```python
from build123d import *

# Parameters (mm, degrees)
IZIM1_W                               = 47
IZIM1_H                               = 96.3
Y_KSEKLIK_EKSTR_ZYON1_DEPTH           = 2
KES_EKSTR_ZYON1_DEPTH                 = 68.315841375
IZIM3_R                               = 3
Y_KSEKLIK_EKSTR_ZYON2_DEPTH           = 5
Y_KSEKLIK_EKSTR_ZYON3_DEPTH           = 2
Y_KSEKLIK_EKSTR_ZYON3_DRAFT           = 4
Y_KSEKLIK_EKSTR_ZYON3_PROFILE_2_DEPTH = 2
Y_KSEKLIK_EKSTR_ZYON3_PROFILE_2_DRAFT = 4
Y_KSEKLIK_EKSTR_ZYON3_PROFILE_3_DEPTH = 2
Y_KSEKLIK_EKSTR_ZYON3_PROFILE_3_DRAFT = 4
IZIM5_W                               = 47
IZIM5_H                               = 2.496748802
KES_EKSTR_ZYON3_DEPTH                 = 4
IZIM6_W                               = 4
IZIM6_H                               = 4
Y_KSEKLIK_EKSTR_ZYON4_DEPTH           = 6
IZIM7_R                               = 1.25
KES_EKSTR_ZYON4_DEPTH                 = 4
KES_EKSTR_ZYON4_DRAFT                 = -2
KES_EKSTR_ZYON4_PROFILE_2_DEPTH       = 4
KES_EKSTR_ZYON4_PROFILE_2_DRAFT       = -2
IZIM8_R                               = 1.25
Y_KSEKLIK_EKSTR_ZYON5_DEPTH           = 0.1
KUBBE5_FACE_RADIUS                    = 1.25
KUBBE5_HEIGHT                         = 1
AYNALAMA8_COPY_1_FACE_RADIUS          = 1.25
AYNALAMA8_COPY_1_HEIGHT               = 1


with BuildPart() as part:
    # Çizim1 → Yükseklik-Ekstrüzyon1 (new body)
    with BuildSketch(Plane(origin=(0, 0, 0), x_dir=(1, 0, 0), z_dir=(0, 1, 0))):
        Rectangle(IZIM1_W, IZIM1_H)
    extrude(amount=Y_KSEKLIK_EKSTR_ZYON1_DEPTH)

    # Çizim2 → Kes-Ekstrüzyon1 (cut, through all)
    with BuildSketch(Plane.ZY.offset(23.5)):
        Polygon((48.15, 0), (43.722619458, 2), (48.15, 2), align=None)
    extrude(amount=-KES_EKSTR_ZYON1_DEPTH, mode=Mode.SUBTRACT)

    # Çizim3 → Yükseklik-Ekstrüzyon2 (add)
    # profile 1 of 4: a face of its own
    with BuildSketch(Plane(origin=(0, 2, 0), x_dir=(1, 0, 0), z_dir=(0, 1, 0))):
        with Locations(Location((-15, 25.194528994, 0), (0, 0, 270))):
            Circle(IZIM3_R)
        with BuildLine():
            ThreePointArc((-16.5, 25.194528994), (-15, 23.694528994), (-13.5, 25.194528994))
            ThreePointArc((-13.5, 25.194528994), (-15, 26.694528994), (-16.5, 25.194528994))
        make_face(mode=Mode.SUBTRACT)
    # profile 2 of 4: a face of its own
    with BuildSketch(Plane(origin=(0, 2, 0), x_dir=(1, 0, 0), z_dir=(0, 1, 0))):
        with Locations(Location((15, 25.194528994, 0), (0, 0, 270))):
            Circle(IZIM3_R)
        with BuildLine():
            ThreePointArc((13.5, 25.194528994), (15, 23.694528994), (16.5, 25.194528994))
            ThreePointArc((16.5, 25.194528994), (15, 26.694528994), (13.5, 25.194528994))
        make_face(mode=Mode.SUBTRACT)
    # profile 3 of 4: a face of its own
    with BuildSketch(Plane(origin=(0, 2, 0), x_dir=(1, 0, 0), z_dir=(0, 1, 0))):
        with Locations(Location((-3.3, -16.805471006, 0), (0, 0, 270))):
            Circle(IZIM3_R)
        with BuildLine():
            ThreePointArc((-1.8, -16.805471006), (-3.3, -15.305471006), (-4.8, -16.805471006))
            ThreePointArc((-4.8, -16.805471006), (-3.3, -18.305471006), (-1.8, -16.805471006))
        make_face(mode=Mode.SUBTRACT)
    # profile 4 of 4: a face of its own
    with BuildSketch(Plane(origin=(0, 2, 0), x_dir=(1, 0, 0), z_dir=(0, 1, 0))):
        with Locations(Location((11.7, -16.805471006, 0), (0, 0, 270))):
            Circle(IZIM3_R)
        with BuildLine():
            ThreePointArc((10.2, -16.805471006), (11.7, -18.305471006), (13.2, -16.805471006))
            ThreePointArc((13.2, -16.805471006), (11.7, -15.305471006), (10.2, -16.805471006))
        make_face(mode=Mode.SUBTRACT)
    extrude(amount=Y_KSEKLIK_EKSTR_ZYON2_DEPTH)


with BuildPart() as y_kseklik_ekstr_zyon3_tool:
    # Çizim4 → Yükseklik-Ekstrüzyon3 (with draft: the straight prism first)
    with BuildSketch(Plane(origin=(0, 18.064663731, 8.160429654), x_dir=(1, 0, 0), z_dir=(0, 0.9113290688724396, 0.4116786710871625))):
        Polygon((20.223356646, -43.072925072), (18.923356646, -43.072925072), (19.573356646, -44.562410878), align=None)
    extrude(amount=Y_KSEKLIK_EKSTR_ZYON3_DEPTH)
    # Yükseklik-Ekstrüzyon3: the draft: its side faces are tilted about the plane it starts from
    y_kseklik_ekstr_zyon3_sides = [y_kseklik_ekstr_zyon3_tool.faces().sort_by_distance(p)[0] for p in [
        (19.573356646, 1.243788246, 47.825717025),
        (19.248356646, 0.937193478, 48.504422881),
        (19.898356646, 0.937193478, 48.504422881),
    ]]
    draft(y_kseklik_ekstr_zyon3_sides, Plane(origin=(0, 18.064663731, 8.160429654), x_dir=(1, 0, 0), z_dir=(0, 0.9113290688724396, 0.4116786710871625)), Y_KSEKLIK_EKSTR_ZYON3_DRAFT)


with BuildPart() as part_1:
    add(part.part)

    # Yükseklik-Ekstrüzyon3: add y_kseklik_ekstr_zyon3_tool
    add(y_kseklik_ekstr_zyon3_tool.part)


with BuildPart() as y_kseklik_ekstr_zyon3_profile_2_tool:
    # Çizim4 → Yükseklik-Ekstrüzyon3 profile 2 (with draft: the straight prism first)
    with BuildSketch(Plane(origin=(0, 18.064663731, 8.160429654), x_dir=(1, 0, 0), z_dir=(0, 0.9113290688724396, 0.4116786710871625))):
        Polygon((0.223356646, -43.072925072), (-1.076643354, -43.072925072), (-0.426643354, -44.562410878), align=None)
    extrude(amount=Y_KSEKLIK_EKSTR_ZYON3_PROFILE_2_DEPTH)
    # Yükseklik-Ekstrüzyon3 profile 2: the draft: its side faces are tilted about the plane it starts from
    y_kseklik_ekstr_zyon3_profile_2_sides = [y_kseklik_ekstr_zyon3_profile_2_tool.faces().sort_by_distance(p)[0] for p in [
        (-0.426643354, 1.243788246, 47.825717025),
        (-0.751643354, 0.937193478, 48.504422881),
        (-0.101643354, 0.937193478, 48.504422881),
    ]]
    draft(y_kseklik_ekstr_zyon3_profile_2_sides, Plane(origin=(0, 18.064663731, 8.160429654), x_dir=(1, 0, 0), z_dir=(0, 0.9113290688724396, 0.4116786710871625)), Y_KSEKLIK_EKSTR_ZYON3_PROFILE_2_DRAFT)


with BuildPart() as part_2:
    add(part_1.part)

    # Yükseklik-Ekstrüzyon3 profile 2: add y_kseklik_ekstr_zyon3_profile_2_tool
    add(y_kseklik_ekstr_zyon3_profile_2_tool.part)


with BuildPart() as y_kseklik_ekstr_zyon3_profile_3_tool:
    # Çizim4 → Yükseklik-Ekstrüzyon3 profile 3 (with draft: the straight prism first)
    with BuildSketch(Plane(origin=(0, 18.064663731, 8.160429654), x_dir=(1, 0, 0), z_dir=(0, 0.9113290688724396, 0.4116786710871625))):
        Polygon((-21.076643354, -43.072925072), (-20.426643354, -44.562410878), (-19.776643354, -43.072925072), align=None)
    extrude(amount=Y_KSEKLIK_EKSTR_ZYON3_PROFILE_3_DEPTH)
    # Yükseklik-Ekstrüzyon3 profile 3: the draft: its side faces are tilted about the plane it starts from
    y_kseklik_ekstr_zyon3_profile_3_sides = [y_kseklik_ekstr_zyon3_profile_3_tool.faces().sort_by_distance(p)[0] for p in [
        (-20.751643354, 0.937193478, 48.504422881),
        (-20.101643354, 0.937193478, 48.504422881),
        (-20.426643354, 1.243788246, 47.825717025),
    ]]
    draft(y_kseklik_ekstr_zyon3_profile_3_sides, Plane(origin=(0, 18.064663731, 8.160429654), x_dir=(1, 0, 0), z_dir=(0, 0.9113290688724396, 0.4116786710871625)), Y_KSEKLIK_EKSTR_ZYON3_PROFILE_3_DRAFT)


with BuildPart() as part_3:
    add(part_2.part)

    # Yükseklik-Ekstrüzyon3 profile 3: add y_kseklik_ekstr_zyon3_profile_3_tool
    add(y_kseklik_ekstr_zyon3_profile_3_tool.part)

    # Çizim5 → Kes-Ekstrüzyon3 (cut)
    with BuildSketch(Plane.XZ):
        with Locations((0, 49.398374401)):
            Rectangle(IZIM5_W, IZIM5_H)
    extrude(amount=KES_EKSTR_ZYON3_DEPTH, mode=Mode.SUBTRACT)

    # Çizim6 → Yükseklik-Ekstrüzyon4 (add)
    with BuildSketch(Plane(origin=(0, 2, 0), x_dir=(1, 0, 0), z_dir=(0, 1, 0))):
        with Locations((-21.5, 46.15)):
            Rectangle(IZIM6_W, IZIM6_H)
        with Locations((21.5, 46.15)):
            Rectangle(IZIM6_W, IZIM6_H)
        with Locations((-21.5, -23.85)):
            Rectangle(IZIM6_W, IZIM6_H)
        with Locations((21.5, -23.85)):
            Rectangle(IZIM6_W, IZIM6_H)
    extrude(amount=Y_KSEKLIK_EKSTR_ZYON4_DEPTH)


with BuildPart() as kes_ekstr_zyon4_tool:
    # Çizim7 → Kes-Ekstrüzyon4 (with draft: the straight prism first)
    with BuildSketch(Plane(origin=(0, 0, -48.15), x_dir=(-1, 0, 0), z_dir=(0, 0, -1))):
        with Locations((-21.5, 6)):
            Circle(IZIM7_R)
    extrude(amount=-KES_EKSTR_ZYON4_DEPTH)
    # Kes-Ekstrüzyon4: the draft: its side faces are tilted about the plane it starts from
    kes_ekstr_zyon4_sides = [kes_ekstr_zyon4_tool.faces().sort_by_distance(p)[0] for p in [
        (22.75, 6, -46.15),
    ]]
    draft(kes_ekstr_zyon4_sides, Plane(origin=(0, 0, -48.15), x_dir=(-1, 0, 0), z_dir=(0, 0, -1)), KES_EKSTR_ZYON4_DRAFT)


with BuildPart() as part_4:
    add(part_3.part)

    # Kes-Ekstrüzyon4: cut by kes_ekstr_zyon4_tool
    add(kes_ekstr_zyon4_tool.part, mode=Mode.SUBTRACT)


with BuildPart() as kes_ekstr_zyon4_profile_2_tool:
    # Çizim7 → Kes-Ekstrüzyon4 profile 2 (with draft: the straight prism first)
    with BuildSketch(Plane(origin=(0, 0, -48.15), x_dir=(-1, 0, 0), z_dir=(0, 0, -1))):
        with Locations((21.5, 6)):
            Circle(IZIM7_R)
    extrude(amount=-KES_EKSTR_ZYON4_PROFILE_2_DEPTH)
    # Kes-Ekstrüzyon4 profile 2: the draft: its side faces are tilted about the plane it starts from
    kes_ekstr_zyon4_profile_2_sides = [kes_ekstr_zyon4_profile_2_tool.faces().sort_by_distance(p)[0] for p in [
        (-20.25, 6, -46.15),
    ]]
    draft(kes_ekstr_zyon4_profile_2_sides, Plane(origin=(0, 0, -48.15), x_dir=(-1, 0, 0), z_dir=(0, 0, -1)), KES_EKSTR_ZYON4_PROFILE_2_DRAFT)


with BuildPart() as part_5:
    add(part_4.part)

    # Kes-Ekstrüzyon4 profile 2: cut by kes_ekstr_zyon4_profile_2_tool
    add(kes_ekstr_zyon4_profile_2_tool.part, mode=Mode.SUBTRACT)

    # Çizim8 → Yükseklik-Ekstrüzyon5 (add)
    with BuildSketch(Plane.ZY.offset(23.5)):
        with Locations(Location((23.85, 6, 0), (0, 0, 180))):
            Circle(IZIM8_R)
    y_kseklik_ekstr_zyon5 = extrude(amount=Y_KSEKLIK_EKSTR_ZYON5_DEPTH)

    # Kubbe5: a dome of height H over a round flat face of radius A is a cap of a sphere of radius (A * A + H * H) / (2 * H)
    kubbe5_r = (KUBBE5_FACE_RADIUS * KUBBE5_FACE_RADIUS + KUBBE5_HEIGHT * KUBBE5_HEIGHT) / (2 * KUBBE5_HEIGHT)
    kubbe5_base = Plane((-23.6, 6, 23.85), z_dir=(-1, 0, 0))
    with Locations(kubbe5_base.offset(KUBBE5_HEIGHT - kubbe5_r)):
        kubbe5_ball = Sphere(kubbe5_r, mode=Mode.PRIVATE)
    add(split(kubbe5_ball, bisect_by=kubbe5_base, keep=Keep.TOP, mode=Mode.PRIVATE))

    # Aynalama8: Yükseklik-Ekstrüzyon5 across plane
    add(y_kseklik_ekstr_zyon5.mirror(Plane(origin=(0, 0, 0), x_dir=(0, 0, 1), z_dir=(1, 0, 0))))

    # Aynalama8 copy 1: a dome of height H over a round flat face of radius A is a cap of a sphere of radius (A * A + H * H) / (2 * H)
    aynalama8_copy_1_r = (AYNALAMA8_COPY_1_FACE_RADIUS * AYNALAMA8_COPY_1_FACE_RADIUS + AYNALAMA8_COPY_1_HEIGHT * AYNALAMA8_COPY_1_HEIGHT) / (2 * AYNALAMA8_COPY_1_HEIGHT)
    aynalama8_copy_1_base = Plane((23.6, 6, 23.85), z_dir=(1, 0, 0))
    with Locations(aynalama8_copy_1_base.offset(AYNALAMA8_COPY_1_HEIGHT - aynalama8_copy_1_r)):
        aynalama8_copy_1_ball = Sphere(aynalama8_copy_1_r, mode=Mode.PRIVATE)
    add(split(aynalama8_copy_1_ball, bisect_by=aynalama8_copy_1_base, keep=Keep.TOP, mode=Mode.PRIVATE))


solid = part_5.part
```
Here's how the part is built. I have some questions about the finished solid (model axes, mm). A direction names the side the tool comes from. Coordinates: 2 decimals unless noted, no trailing zeros. Order: outer loops, then holes, each group sorted by start corner. A loop starts at its lowest first (then second) coordinate and runs counter-clockwise, first axis right, second up. Notation, with made-up numbers: M -33,88 L 26,88 A19 ccw 26,108 Z; hole C 19.5,18.5 d7. An arc over 180 degrees is marked long. Answer as a JSON object with one key per item and string values. Group by question number.
(1) Which directions (+Z, -Z, +X, -X, +Y, -Y) give clear straight access to the entire face, cutting with the end or side of a thin tool? Please do faces 1 (the face through (-3.105, 4.465, 18.293)), 2 (the face through (-22, 5, 21.85)), 3 (the face through (11, 7, 15)).
(2) Suppose I cut it at A-A, the plane x = 21.5. Please give me the cut outline in (y, z), then the cut area to 3 significant figures.
(3) Suppose I cut it at B-B, the plane z = -2. Please give me the cut outline in (x, y).
(4) If we mould it in two halves opening along Z, with no side actions, what happens to faces 4 (the face through (-20.16, 0.94, 48.46)), 5 (the face through (-16, 7, -27)), 6 (the face through (0, 1, -48.15)), 7 (the face through (21, 5, 21.85))? For each: released by +Z, released by -Z, zero draft, split by the parting line, or undercut.
(5) I need wall thicknesses on probe 1 along X at (y, z) = (4.5, 17); probe 2 along Y at (x, z) = (1.5, 42.5); probe 3 along X at (y, z) = (0.75, -5). Which ranges of each line are inside material? Lowest first, please.
(6) For pin 1 (3 mm diameter, centred on x = -21.5, y = 5, fed in from +Z); pin 2 (3 mm diameter, centred on x = 4, z = 6, fed in from +Y); pin 3 (4.5 mm diameter, centred on y = 4, z = -47, fed in from -X), each with a flat end and sliding along its axis, tell me the tip position at first contact or that it passes through.
Values found:
{
 "1": {"face 1": "+Y", "face 2": "+X, -X, +Y", "face 3": "+Z, -Z, +X, -X, +Y"},
 "2": {"outline": "M 0,-48.15 L 4.75,-48.15 L 4.89,-44.15 L 2,-44.15 L 2,21.85 L 8,21.85 L 8,25.85 L 2,25.85 L 2,43.72 L 0,48.15 Z; M 7.11,-44.15 L 7.25,-48.15 L 8,-48.15 L 8,-44.15 Z", "area": "227 mm^2"},
 "3": {"outline": "M -23.5,0 L 23.5,0 L 23.5,2 L -23.5,2 Z"},
 "4": {"face 4": "released by +Z", "face 5": "zero draft", "face 6": "released by -Z", "face 7": "undercut"},
 "5": {"probe 1": "x = -6.29 to -4.79, -1.81 to -0.31, 8.71 to 10.21, 13.19 to 14.69", "probe 2": "y = 0 to 2", "probe 3": "x = -23.5 to 23.5"},
 "6": {"pin 1": "stops at z = 25.85", "pin 2": "stops at y = 2", "pin 3": "stops at x = -23.5"}
}
